Print and shaded views of the part. All mm, measured from the part's lowest x, y and z. A direction names the side the tool comes from. Give positions to 0.01 mm unless a question says otherwise; leave off trailing zeros. Order: outer loops, then holes, each group sorted by start corner. A loop starts at its lowest first (then second) coordinate and runs counter-clockwise, first axis right, second up. Notation, with made-up numbers: (57.25, 52.5) -> (81.25, 52.5) arc R16 cw to (81.25, 73.5) -> close; hole circle Ø5 at (38.5, -23). An arc over 180 degrees is marked (long way). One line per question, with ' | ' between items. Start each with the question number.
(1) Pin check, flat tips, straight feed: pin 1 Ø10 at (x, z) = (37.5, 144) entering from +Y (3 decimals); pin 2 Ø2 at (x, y) = (44, 39.5) entering from -Z; pin 3 Ø3 at (x, z) = (28.5, 54) entering from -Y; pin 4 Ø12 at (y, z) = (38.5, 30) entering from -X (3 decimals). Stop position of each tip, or through.
(2) Which spindle directions (+Z, -Z, +X, -X, +Y, -Y) get a long thin tool onto all of the face, cutting with end or side? Do the marked faces 1 and 2. Say none if no direction does.
(3) Cut at A-A (z = 152.4). Give the cut face in (x, y) (1 decimal).
(4) Drill centre lines: L1, parallel to X at y = 3, z = 25; L2, parallel to Y at x = 10, z = 116 (1 decimal); L3, parallel to X at y = 34, z = 51 (1 decimal). Where is each one in solid material? Low to high. Write a range as from..to.
(5) Cut at D-D (y = 17). Give the cut face in (x, z) (1 decimal).
(6) Cut at C-C (x = 41.5). Give the cut face in (y, z) (1 decimal), then the cut area to 3 significant figures.
(7) Cut at B-B (z = 67.5). Give the cut face in (x, y) (1 decimal).
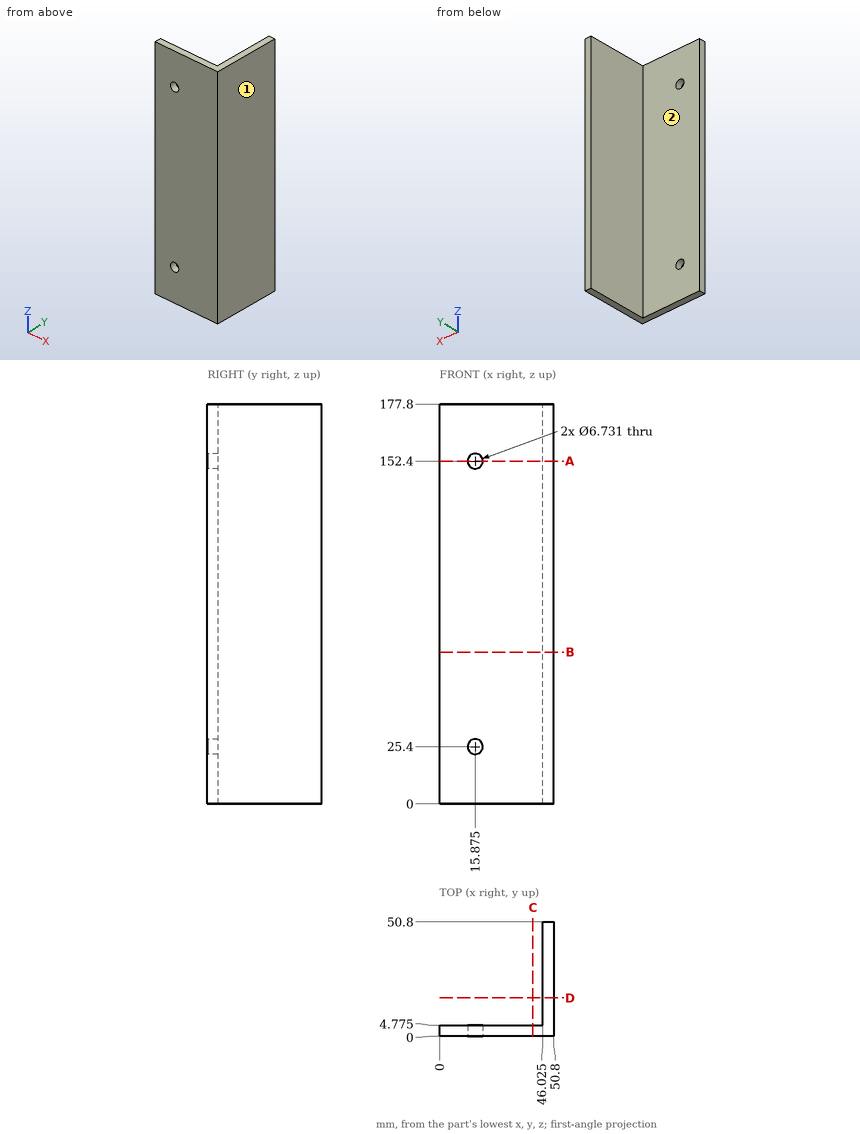
Result set:
1) pin 1: stops at y = 4.775 | pin 2: passes through | pin 3: stops at y = 0 | pin 4: stops at x = 46.025
2) face 1: +Z, -Z, +X, +Y, -Y | face 2: +Z, -Z, -X, +Y
3) outline: (0, 0) -> (12.5, 0) -> (12.5, 4.8) -> (0, 4.8) -> close; (19.2, 0) -> (50.8, 0) -> (50.8, 50.8) -> (46, 50.8) -> (46, 4.8) -> (19.2, 4.8) -> close
4) L1: x = 0..12.53, 19.22..50.8 | L2: y = 0..4.8 | L3: x = 46..50.8
5) outline: (46, 0) -> (50.8, 0) -> (50.8, 177.8) -> (46, 177.8) -> close
6) outline: (0, 0) -> (4.8, 0) -> (4.8, 177.8) -> (0, 177.8) -> close | area: 849 mm2
7) outline: (0, 0) -> (50.8, 0) -> (50.8, 50.8) -> (46, 50.8) -> (46, 4.8) -> (0, 4.8) -> close
